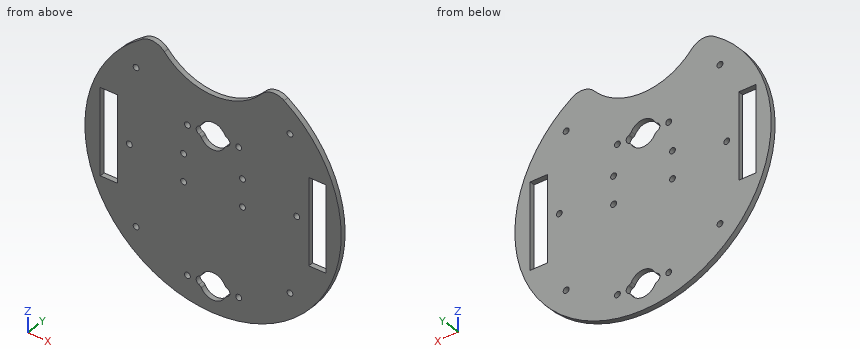
from build123d import *

# Parameters (mm, degrees)
SKETCH1_R           = 75
BOSS_EXTRUDE1_DEPTH = 3
SKETCH2_W           = 10
SKETCH2_H           = 50
CUT_EXTRUDE1_DEPTH  = 6.35
CUT_EXTRUDE2_DEPTH  = 10
CUT_EXTRUDE3_DEPTH  = 10
FILLET2_R           = 10
SKETCH7_R           = 1.7145
CUT_EXTRUDE5_DEPTH  = 3
SKETCH6_R           = 1.7145
CUT_EXTRUDE6_DEPTH  = 3
FILLET4_R           = 3
SKETCH8_R           = 1.7145
CUT_EXTRUDE7_DEPTH  = 4.0000001


with BuildPart() as part:
    # Sketch1 → Boss-Extrude1 (new body)
    with BuildSketch(Plane(origin=(0, 0, 0), x_dir=(1, 0, 0), z_dir=(0, 1, 0))):
        Circle(SKETCH1_R)
    extrude(amount=BOSS_EXTRUDE1_DEPTH)

    # Sketch2 → Cut-Extrude1 (cut)
    with BuildSketch(Plane(origin=(0, 3, 0), x_dir=(1, 0, 0), z_dir=(0, 1, 0))):
        with Locations((-61, 0)):
            Rectangle(SKETCH2_W, SKETCH2_H)
        with Locations((61, 0)):
            Rectangle(SKETCH2_W, SKETCH2_H)
    extrude(amount=-CUT_EXTRUDE1_DEPTH, mode=Mode.SUBTRACT)

    # Sketch3 → Cut-Extrude2 (cut)
    with BuildSketch(Plane(origin=(0, 3, 0), x_dir=(1, 0, 0), z_dir=(0, 1, 0))):
        with BuildLine():
            ThreePointArc((-7.335762693, -27.499817134), (0, -32.75), (7.335762693, -27.499817134))
            ThreePointArc((7.335762693, -27.499817134), (9.866, -25), (7.335762693, -22.500182866))
            ThreePointArc((7.335762693, -22.500182866), (0, -17.25), (-7.335762693, -22.500182866))
            ThreePointArc((-7.335762693, -22.500182866), (-9.866, -25), (-7.335762693, -27.499817134))
        make_face()
        with BuildLine():
            ThreePointArc((-7.335762693, 62.499817134), (-9.866, 60), (-7.335762693, 57.500182866))
            ThreePointArc((-7.335762693, 57.500182866), (0, 52.25), (7.335762693, 57.500182866))
            ThreePointArc((7.335762693, 57.500182866), (9.866, 60), (7.335762693, 62.499817134))
            ThreePointArc((7.335762693, 62.499817134), (0, 67.75), (-7.335762693, 62.499817134))
        make_face()
    extrude(amount=-CUT_EXTRUDE2_DEPTH, mode=Mode.SUBTRACT)

    # Sketch4 → Cut-Extrude3 (cut)
    with BuildSketch(Plane(origin=(0, 3, 0), x_dir=(1, 0, 0), z_dir=(0, 1, 0))):
        with BuildLine():
            ThreePointArc((-33.160552015, -67.270928268), (0, -47.932265908), (33.160552015, -67.270928268))
            ThreePointArc((33.160552015, -67.270928268), (0, -75), (-33.160552015, -67.270928268))
        make_face()
    extrude(amount=-CUT_EXTRUDE3_DEPTH, mode=Mode.SUBTRACT)

    # Fillet2
    fillet2_edges = [part.edges().sort_by_distance(p)[0] for p in [
        (-33.160552015, 1.5, 67.270928268),
        (33.160552015, 1.5, 67.270928268),
    ]]
    fillet(fillet2_edges, radius=FILLET2_R)

    # Sketch7 → Cut-Extrude5 (cut)
    with BuildSketch(Plane(origin=(0, 3, 0), x_dir=(1, 0, 0), z_dir=(0, 1, 0))):
        with Locations((-48.975, 0)):
            Circle(SKETCH7_R)
        with Locations((-17.225, 7.9375)):
            Circle(SKETCH7_R)
        with Locations((-17.225, -7.9375)):
            Circle(SKETCH7_R)
        with Locations((17.225, -7.9375)):
            Circle(SKETCH7_R)
        with Locations((17.225, 7.9375)):
            Circle(SKETCH7_R)
        with Locations((48.975, 0)):
            Circle(SKETCH7_R)
    extrude(amount=-CUT_EXTRUDE5_DEPTH, mode=Mode.SUBTRACT)

    # Sketch6 → Cut-Extrude6 (cut)
    with BuildSketch(Plane(origin=(0, 3, 0), x_dir=(1, 0, 0), z_dir=(0, 1, 0))):
        with Locations((-15, 60)):
            Circle(SKETCH6_R)
        with Locations((15, 60)):
            Circle(SKETCH6_R)
        with Locations((-15, -25)):
            Circle(SKETCH6_R)
        with Locations((15, -25)):
            Circle(SKETCH6_R)
    extrude(amount=-CUT_EXTRUDE6_DEPTH, mode=Mode.SUBTRACT)

    # Fillet4
    fillet4_edges = [part.edges().sort_by_distance(p)[0] for p in [
        (-7.335762693, 1.5, -62.499817134),
        (7.335762693, 1.5, -62.499817134),
        (7.335762693, 1.5, -57.500182866),
        (-7.335762693, 1.5, -57.500182866),
        (7.335762693, 1.5, 22.500182866),
        (7.335762693, 1.5, 27.499817134),
        (-7.335762693, 1.5, 27.499817134),
        (-7.335762693, 1.5, 22.500182866),
    ]]
    fillet(fillet4_edges, radius=FILLET4_R)

    # Sketch8 → Cut-Extrude7 (cut, through all)
    with BuildSketch(Plane(origin=(0, 3, 0), x_dir=(1, 0, 0), z_dir=(0, 1, 0))):
        with Locations((-45, 45)):
            Circle(SKETCH8_R)
        with Locations((45, 45)):
            Circle(SKETCH8_R)
        with Locations((45, -45)):
            Circle(SKETCH8_R)
        with Locations((-45, -45)):
            Circle(SKETCH8_R)
    extrude(amount=-CUT_EXTRUDE7_DEPTH, mode=Mode.SUBTRACT)


solid = part.part
Read the model definition and answer for the solid it produces. Units are mm, in the model's axes. Coordinates: 2 decimals unless noted, no trailing zeros. Order: outer loops, then holes, each group sorted by start corner. A loop starts at its lowest first (then second) coordinate and runs counter-clockwise, first axis right, second up. Notation, with made-up numbers: (-28.5, 46) -> (25.5, 46) arc R29 cw to (25.5, 71) -> close; hole circle Ø11 at (33, 37.5). An arc over 180 degrees is marked (long way). Answer as a JSON object with one key per item and string values.
1) Consider line 1 along X through (y, z) = (1.35, 0); line 2 along X through (y, z) = (1.6, -60); line 3 along X through (y, z) = (2.3, -45). Determine where each line is inside the solid, lowest interval first. Write a range as from..to.
Model answer:
{"line 1": "x = -75..-66, -56..-50.69, -47.26..47.26, 50.69..56, 66..75", "line 2": "x = -45..-16.71, -13.29..-9.87, 9.87..13.29, 16.71..45", "line 3": "x = -60..-46.71, -43.29..43.29, 46.71..60"}
2) A cutting plane is placed at A-A, the plane x = 0. Determine the outline of the cut face in (y, z).
Model answer:
{"outline": "(0, -75) -> (3, -75) -> (3, -67.75) -> (0, -67.75) -> close; (0, -52.25) -> (3, -52.25) -> (3, 17.25) -> (0, 17.25) -> close; (0, 32.75) -> (3, 32.75) -> (3, 47.93) -> (0, 47.93) -> close"}
3) A cutting plane is placed at B-B, the plane z = 0. Determine the outline of the cut face in (x, y), plus the area to 3 significant figures.
Model answer:
{"outline": "(-75, 0) -> (-66, 0) -> (-66, 3) -> (-75, 3) -> close; (-56, 0) -> (-50.69, 0) -> (-50.69, 3) -> (-56, 3) -> close; (-47.26, 0) -> (47.26, 0) -> (47.26, 3) -> (-47.26, 3) -> close; (50.69, 0) -> (56, 0) -> (56, 3) -> (50.69, 3) -> close; (66, 0) -> (75, 0) -> (75, 3) -> (66, 3) -> close", "area": "369 mm²"}
4) A cutting plane is placed at C-C, the plane x = 45. Determine the outline of the cut face in (y, z), plus the area to 3 significant figures.
Model answer:
{"outline": "(0, -60) -> (3, -60) -> (3, -46.71) -> (0, -46.71) -> close; (0, -43.29) -> (3, -43.29) -> (3, 43.29) -> (0, 43.29) -> close; (0, 46.71) -> (3, 46.71) -> (3, 60) -> (0, 60) -> close", "area": "339 mm²"}
5) Each of these flat-tipped pins is pushed along its axis until it touches: pin 1 (3 mm diameter, centred on x = -17.23, z = -7.94, fed in from -Y); pin 2 (0.9 mm diameter, centred on y = 1, z = -5, fed in from -X); pin 3 (1.5 mm diameter, centred on y = 1, z = 6.5, fed in from +X). Where does it stop, or does it pass through?
Model answer:
{"pin 1": "passes through", "pin 2": "stops at x = -74.86", "pin 3": "stops at x = 74.78"}
6) A cutting plane is placed at D-D, the plane y = 2.3. State how many separate pieces and enclosed holes the cut face has, plus the area to 3 significant figures.
Model answer:
{"separate pieces": "1", "enclosed holes": "18", "area": "14,800 mm²"}
